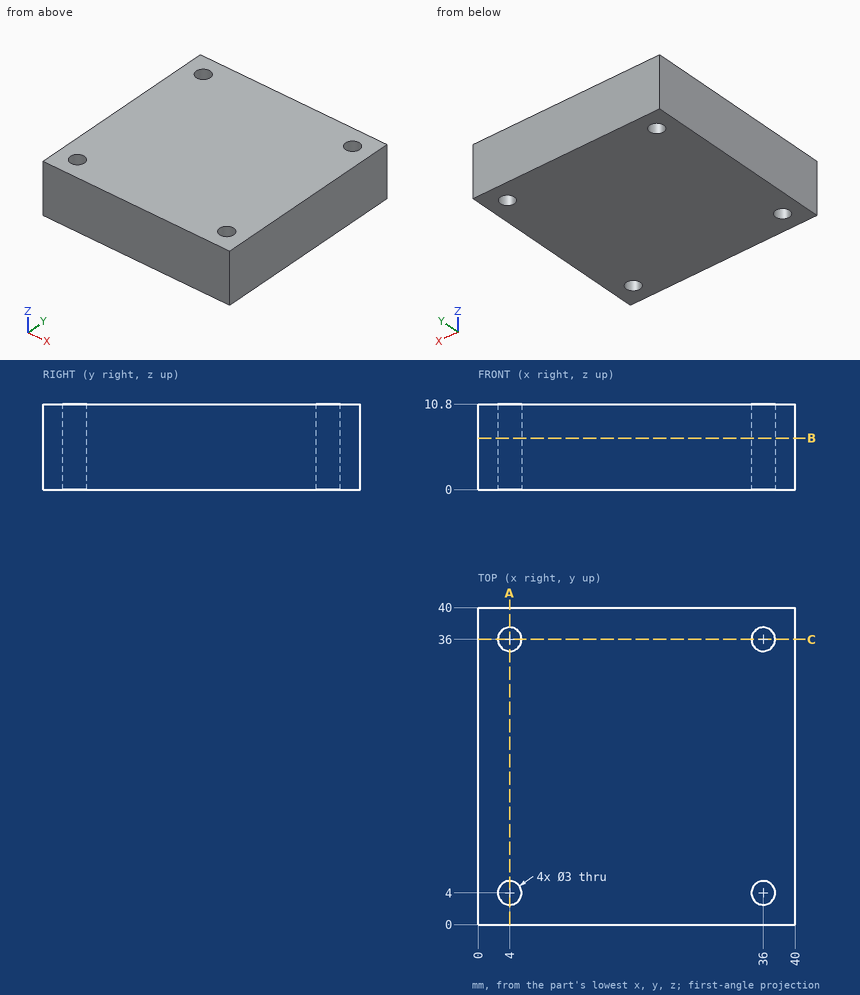
Design review of the part shown in the three views and the two pictorial views. Dimensions are in mm from the part's minimum x, y and z. Round coordinates to 2 decimals unless told otherwise and drop trailing zeros. Order: outer loops, then holes, each group sorted by start corner. A loop starts at its lowest first (then second) coordinate and runs counter-clockwise, first axis right, second up.
(1) For P1, Ø2.5, axis at x = 36, y = 36, coming from the -Z side, flat-tipped, find the tip position at first contact; note if it passes through.
Working result:
P1: passes through
(2) Take a section at B-B, the plane z = 6.5. State the section outline as (x, y) points, plus the area to 3 significant figures.
Working result:
outline: (0, 0) - (40, 0) - (40, 40) - (0, 40) - close; hole circle Ø3 at (4, 4); hole circle Ø3 at (4, 36); hole circle Ø3 at (36, 4); hole circle Ø3 at (36, 36)
area: 1,570 mm2
(3) Take a section at A-A, the plane x = 4. State the section outline as (y, z) points.
Working result:
outline: (0, 0) - (2.5, 0) - (2.5, 10.8) - (0, 10.8) - close; (5.5, 0) - (34.5, 0) - (34.5, 10.8) - (5.5, 10.8) - close; (37.5, 0) - (40, 0) - (40, 10.8) - (37.5, 10.8) - close
(4) Wall thickness on L1, parallel to Y at x = 4, z = 3.75; L2, parallel to X at y = 35.5, z = 7: over which ranges is each line inside the solid? List them lowest first.
Working result:
L1: y = 0 to 2.5, 5.5 to 34.5, 37.5 to 40
L2: x = 0 to 2.59, 5.41 to 34.59, 37.41 to 40
